```python
from build123d import *

# Parameters (mm, degrees)
F0_R     = 2.5
F0_R_2   = 0.4435
F1_DEPTH = 3.375
F0_R_3   = 3
F2_DEPTH = 1.375
F3_DEPTH = 0.875
F4_SIZE  = 0.25
F5_DEPTH = 1


with BuildPart() as f1:
    # F0 (on Top) → F1 (new body)
    with BuildSketch(Plane.XY):
        Circle(F0_R)
        Circle(F0_R_2, mode=Mode.SUBTRACT)
    extrude(amount=F1_DEPTH)

    # F0 (on Top) → F2 (join)
    with BuildSketch(Plane.XY):
        Circle(F0_R_3)
        Circle(F0_R, mode=Mode.SUBTRACT)
    extrude(amount=F2_DEPTH)

    # F0 (on Top) → F3 (join)
    with BuildSketch(Plane.XY):
        Circle(F0_R_2)
    extrude(amount=F3_DEPTH)

    # F4
    f4_edges = [f1.edges().sort_by_distance(p)[0] for p in [
        (-2.5, 0, 3.375),
    ]]
    chamfer(f4_edges, length=F4_SIZE)

    # F0 (on Top) → F5 (join)
    with BuildSketch(Plane.XY):
        Circle(F0_R_3)
        Circle(F0_R, mode=Mode.SUBTRACT)
        Circle(F0_R)
        Circle(F0_R_2, mode=Mode.SUBTRACT)
        Circle(F0_R_2)
    extrude(amount=-F5_DEPTH)

    # F6 (on Right) → F7 (revolve, cut)
    with BuildSketch(Plane.YZ):
        Polygon((-6.6943974234, 0.9619678603), (-6.6943974234, 0), (-3.1168663409, 0.9619678603), align=None)
    revolve(axis=Axis((0, 0, 0.9346584557), (0, 0, 1)), mode=Mode.SUBTRACT)


solid = f1.part
```
Work out the finished part from the listing and answer in its coordinate system (mm). A direction names the side the tool comes from. Round coordinates to 2 decimals unless told otherwise and drop trailing zeros. Write each loop counter-clockwise with the first axis right and the second up, starting at its lowest first coordinate (ties: lowest second). Pieces come first, ordered by that corner, then holes.
1) Which of the six approach directions +Z, -Z, +X, -X, +Y, -Y give full straight-line access (tool end or side, diameter ignored) to faces 4 (the face through (-3, 0, 0)), 5 (the face through (-0.096, -0.433, 2.108))?
2) A cutting plane is placed at C-C on z = 1.7. Determine the outline of the cut face in (x, y).
3) Flat-ended cylindrical pins translate along their axes: P1, Ø2, axis at x = 1, z = 3, coming from the -Y side; P2, Ø1, axis at y = -1.5, z = 1, coming from the +X side. Find the tip coordinate at first contact, or state that the pin passes through.
4) A cutting plane is placed at D-D on z = 0. Determine the outline of the cut face in (x, y), and give its area (3 significant figures).
5) Determine the mould class of faces 1 (the face through (0, 0, -1)), 2 (the face through (0, 0, 0.875)), 3 (the face through (-0.54, -2.44, 2.24)) for opening direction Y: pulls with the +Y half, pulls with the -Y half, needs draft (parallel to the pull), parting line crosses it, or undercut.
6) Consider probe 1 along Y at (x, z) = (0, 2.55); probe 2 along Z at (x, y) = (2.5, -1.15) (3 decimals); probe 3 along Z at (x, y) = (0.15, 0) (3 decimals). Determine where each line is inside the solid, lowest interval first.
Entries:
1. face 4: +Z, -Z
1. face 5: +Z
2. outline: circle Ø5 at (0, 0); hole circle Ø0.89 at (0, 0)
3. P1: stops at y = -2.5
3. P2: stops at x = 2.83
4. outline: circle Ø6 at (0, 0)
4. area: 28.3 mm2
5. face 1: needs draft
5. face 2: undercut
5. face 3: parting line crosses it
6. probe 1: y = -2.5 to -0.44, 0.44 to 2.5
6. probe 2: z = -1 to 1.375
6. probe 3: z = -1 to 0.875
